Input: dimensioned drawing with shaded views. Units: mm. Origin: part minimum x, y, z. A direction names the side the tool comes from. Round coordinates to 2 decimals unless told otherwise and drop trailing zeros. Loops run counter-clockwise (first coordinate to the right, second up) from the corner with the lowest first, then second, coordinate; pieces in that order, holes last. Notation, with made-up numbers: (36, 35) - (50, 35) arc R21 cw to (50, 49) - close; hole circle Ø6 at (-21.5, 6). An arc over 180 degrees is marked (long way). Answer as a JSON object with one key per item and string values. Group by question number.
Item 1: Section B-B (y = 8.25). Return the cut outline in (x, z).
Item 2: Reachability of the marked faces 4 and 5 from +Z, -Z, +X, -X, +Y, -Y: full face, straight path, thin tool, end or side. Return the list, or none.
Item 3: Section A-A (z = 3). Return the cut outline in (x, y).
Item 4: First-contact query: pin 1 (3 mm diameter, centred on y = 3.5, z = 3, fed in from -X); pin 2 (1 mm diameter, centred on x = 5, z = 5, fed in from -Y); pin 3 (1.3 mm diameter, centred on x = 2.5, z = 3, fed in from +Y). Flat tips, straight axial feed; report the tip coordinate or a pass-through.
Item 5: Line query: line 1 (Y direction, x = 3.8, z = 4.5); line 2 (X direction, y = 11.75, z = 4.3); line 3 (X direction, y = 11.75, z = 1.8). Output: solid intervals per line, ascending.
Item 6: Draft query along Z for the marked faces 1, 2 and 3. Return one class per face: released by +Z, released by -Z, zero draft, split by the parting line, or undercut.
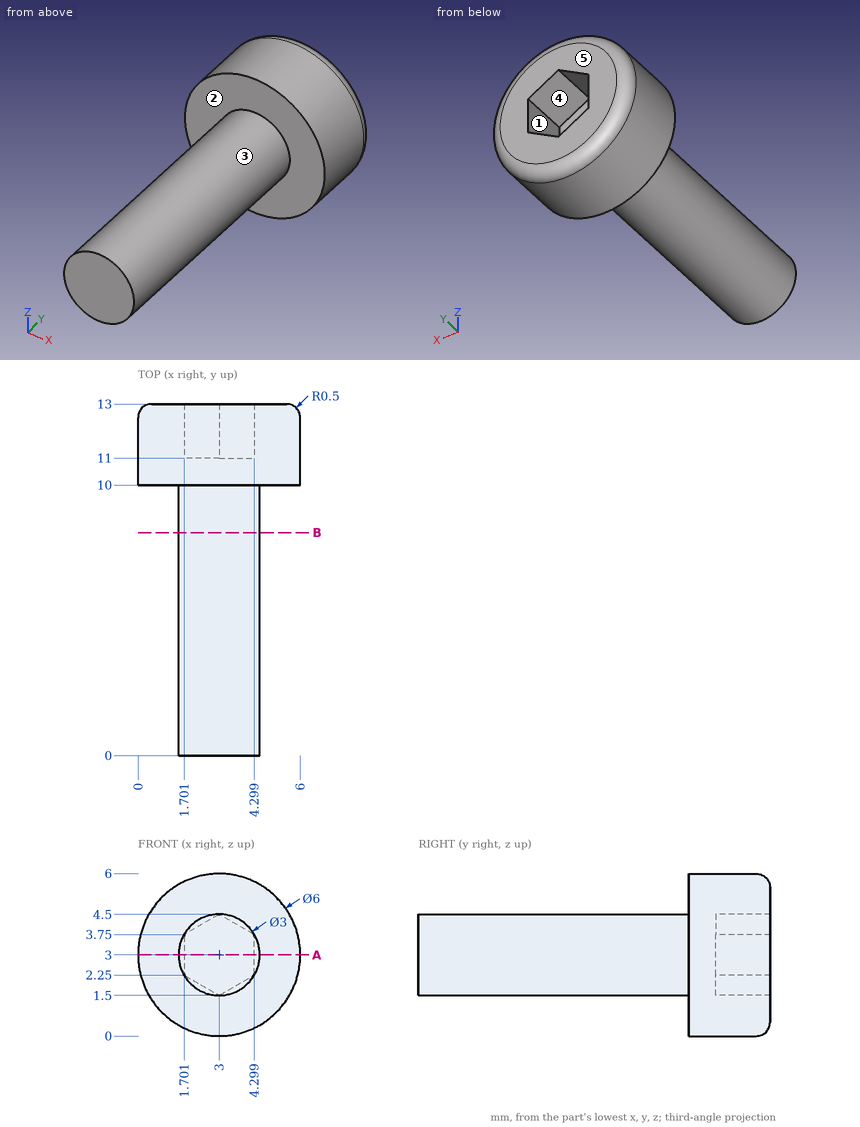
Values:
{
 "1": {"outline": "circle Ø3 at (3, 3)"},
 "2": {"face 4": "+Y", "face 5": "+Z, -Z, +X, -X, +Y"},
 "3": {"outline": "(0, 10) - (1.5, 10) - (1.5, 0) - (4.5, 0) - (4.5, 10) - (6, 10) - (6, 12.5) arc R0.5 ccw to (5.5, 13) - (4.3, 13) - (4.3, 11) - (1.7, 11) - (1.7, 13) - (0.5, 13) arc R0.5 ccw to (0, 12.5) - close"},
 "4": {"pin 1": "stops at x = 1.5", "pin 2": "stops at y = 10", "pin 3": "stops at y = 11"},
 "5": {"line 1": "y = 10 to 13", "line 2": "x = 0.3 to 2.65, 3.35 to 5.7", "line 3": "x = 0.25 to 2.48, 3.52 to 5.75"},
 "6": {"face 1": "undercut", "face 2": "zero draft", "face 3": "split by the parting line"}
}
